```python
from build123d import *

# Parameters (mm, degrees)
BOSS_EXTRUDE1_DEPTH               = 19.05
F_1_4_20_TAPPED_HOLE1_D           = 5.1054
F_1_4_20_TAPPED_HOLE1_DEPTH       = 16.51
F_1_4_20_TAPPED_HOLE1_CSINK_D     = 6.3754
F_1_4_20_TAPPED_HOLE1_CSINK_ANGLE = 90
F_1_4_20_TAPPED_HOLE1_TIP         = 1.533816902
SKETCH3_R                         = 4.7244
CUT_EXTRUDE1_DEPTH                = 4.7244


with BuildPart() as part:
    # Sketch2 → Boss-Extrude1 (new body)
    with BuildSketch(Plane(origin=(0, 0, 0), x_dir=(0, 0, -1), z_dir=(1, 0, 0))):
        with BuildLine():
            Line((0, 0), (50.8, 0))
            Line((50.8, 0), (50.8, 36.83))
            Line((50.8, 36.83), (36.109953655, 36.83))
            ThreePointArc((36.109953655, 36.83), (17.145, 38.1), (36.109953655, 39.37))
            Line((36.109953655, 39.37), (50.8, 39.37))
            Line((50.8, 39.37), (50.8, 76.2))
            Line((50.8, 76.2), (0, 76.2))
            Line((0, 76.2), (0, 0))
        make_face()
    extrude(amount=BOSS_EXTRUDE1_DEPTH)

    # 1/4-20 Tapped Hole1
    with Locations(Plane(origin=(0, 0, 0), x_dir=(-1, 0, 0), z_dir=(0, -1, 0))):
        with Locations((-9.525, 12.7), (-9.525, 38.1)):
            CounterSinkHole(F_1_4_20_TAPPED_HOLE1_D / 2, F_1_4_20_TAPPED_HOLE1_CSINK_D / 2, depth=F_1_4_20_TAPPED_HOLE1_DEPTH, counter_sink_angle=F_1_4_20_TAPPED_HOLE1_CSINK_ANGLE)
            with Locations((0, 0, -(F_1_4_20_TAPPED_HOLE1_DEPTH + F_1_4_20_TAPPED_HOLE1_TIP / 2))):  # 118° drill point
                Cone(0, F_1_4_20_TAPPED_HOLE1_D / 2, F_1_4_20_TAPPED_HOLE1_TIP, mode=Mode.SUBTRACT)

    # Sketch3 → Cut-Extrude1 (cut)
    with BuildSketch(Plane(origin=(0, 76.2, 0), x_dir=(1, 0, 0), z_dir=(0, 1, 0))):
        with Locations((9.525, 31.75)):
            Circle(SKETCH3_R)
    extrude(amount=-CUT_EXTRUDE1_DEPTH, mode=Mode.SUBTRACT)


solid = part.part
```
Work out the finished part from the listing and answer in its coordinate system (mm). A direction names the side the tool comes from. Round coordinates to 2 decimals unless told otherwise and drop trailing zeros. Loops run counter-clockwise (first coordinate to the right, second up) from the corner with the lowest first, then second, coordinate; pieces in that order, holes last.
(1) For faces 1 (the flat face through (9, 58, -50.8)), 2 (the flat face through (9, 71.476, -32)), 3 (the cylindrical face through (9, 8.7, -35.6)), 4 (the flat face through (9, 36.83, -44)), 5 (the flat face through (9, 76.2, -26)), determine the directions among +Z, -Z, +X, -X, +Y, -Y from which every point of the face is accessible in a straight line to the end or side of a thin tool.
Computed values:
face 1: -Z, +X, -X, +Y, -Y
face 2: +Y
face 3: -Y
face 4: -Z, +X, -X
face 5: +Z, -Z, +X, -X, +Y
(2) Find the intervals of material crossed by L1, parallel to X at y = 74.4, z = -31.75; L2, parallel to X at y = 12, z = -13; L3, parallel to Y at x = 5, z = -44, in increasing order.
Computed values:
L1: x = 0 to 4.8, 14.25 to 19.05
L2: x = 0 to 6.99, 12.06 to 19.05
L3: y = 0 to 36.83, 39.37 to 76.2
(3) The mould has two halves that part along X. Classify faces 6 (the flat face through (0, 47, -19)), 7 (the flat face through (9, 39, 0)), 8 (the flat face through (19.05, 47, -19)), 9 (the cylindrical face through (9, 8.7, -10.2)): pulls with the +X half, pulls with the -X half, needs draft (parallel to the pull), parting line crosses it, or undercut.
Computed values:
face 6: pulls with the -X half
face 7: needs draft
face 8: pulls with the +X half
face 9: undercut
(4) The part is cut by section D-D, the plane y = 38.1. Give the vertices of the cut face in (x, z) (3 decimals), and give its area (3 significant figures).
Computed values:
outline: (0, -17.145) - (19.05, -17.145) - (19.05, 0) - (0, 0) - close
area: 327 mm2
(5) The part is cut by section B-B, the plane y = 11.5. Give the vertices of the cut face in (x, z) (3 decimals).
Computed values:
outline: (0, -50.8) - (19.05, -50.8) - (19.05, 0) - (0, 0) - close; hole circle Ø5.105 at (9.525, -38.1); hole circle Ø5.105 at (9.525, -12.7)
(6) The part is cut by section C-C, the plane z = -18. Give the vertices of the cut face in (x, y).
Computed values:
outline: (0, 0) - (19.05, 0) - (19.05, 34.16) - (0, 34.16) - close; (0, 42.04) - (19.05, 42.04) - (19.05, 76.2) - (0, 76.2) - close
(7) The part is cut by section A-A, the plane z = -46. Give the vertices of the cut face in (x, y).
Computed values:
outline: (0, 0) - (19.05, 0) - (19.05, 36.83) - (0, 36.83) - close; (0, 39.37) - (19.05, 39.37) - (19.05, 76.2) - (0, 76.2) - close
